```python
from build123d import *

# Parameters (mm, degrees)
BOSS_EXTRUDE1_DEPTH = 2.5
FILLET1_R           = 6.35


with BuildPart() as part:
    # Sketch1 → Boss-Extrude1 (new, symmetric)
    with BuildSketch(Plane.XY):
        Polygon((-63.5, 0), (-57.15, 25.4), (63.5, 25.4), (63.5, -25.4), (-63.5, -25.4), align=None)
    extrude(amount=BOSS_EXTRUDE1_DEPTH, both=True)

    # Fillet1
    fillet1_edges = [part.edges().sort_by_distance(p)[0] for p in [
        (63.5, -25.4, 0),
        (-63.5, -25.4, 0),
        (-63.5, 0, 0),
        (-57.15, 25.4, 0),
        (63.5, 25.4, 0),
    ]]
    fillet(fillet1_edges, radius=FILLET1_R)


solid = part.part
```
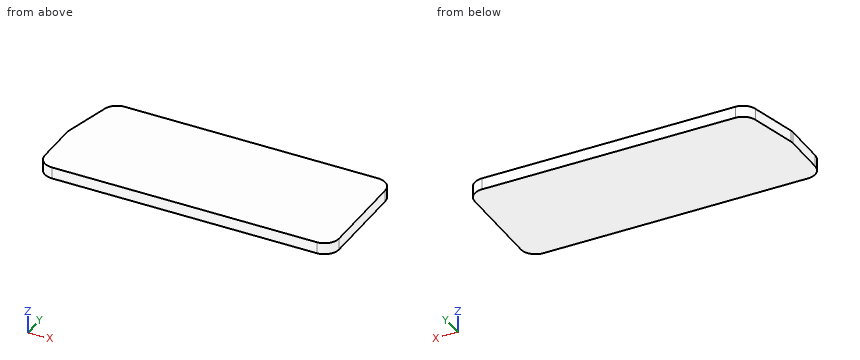
Could you check a few things on this model? Use its own coordinates, in mm. Coordinates: 2 decimals unless noted, no trailing zeros. Write each loop counter-clockwise with the first axis right and the second up, starting at its lowest first coordinate (ties: lowest second). Pieces come first, ordered by that corner, then holes. Notation, with made-up numbers: M -14,30.5 L 45,30.5 A15 cw 45,55.5 Z; hole C -8.75,-21 d10. An arc over 180 degrees is marked long. Answer as CSV lines item,"result". Start each with the question number.
1) Please list where these lines run through material, in increasing order: line 1 (X direction, y = 9.5, z = -0.05) (3 decimals); line 2 (X direction, y = 14, z = 1.75); line 3 (Y direction, x = -57.5, z = -0.7). Write a range as from..to.
2) I want a section at C-C, the plane y = 15.5. Please give me the cut outline in (x, z) (3 decimals).
3) I want a section at B-B, the plane y = 9. Please give me the cut outline in (x, z).
4) For P1, Ø1.5, axis at y = 10, z = -2, coming from the -X side, with a flat end and sliding along its axis, tell me the tip position at first contact or that it passes through.
5) I want a section at A-A, the plane z = 1.75. Please give me the cut outline in (x, y), and give its area (3 significant figures).
Data:
1,line 1,"x = -61.125..63.5"
1,line 2,"x = -60..63.5"
1,line 3,"y = -25.39..22.54"
2,outline,"M -59.625,-2.5 L 63.5,-2.5 L 63.5,2.5 L -59.625,2.5 Z"
3,outline,"M -61.25,-2.5 L 63.5,-2.5 L 63.5,2.5 L -61.25,2.5 Z"
4,P1,"stops at x = -61.19"
5,outline,"M -63.5,-19.05 A6.35 ccw -57.15,-25.4 L 57.15,-25.4 A6.35 ccw 63.5,-19.05 L 63.5,19.05 A6.35 ccw 57.15,25.4 L -52.19,25.4 A6.35 ccw -58.35,20.59 L -63.31,0.76 A6.35 ccw -63.5,-0.78 Z"
5,area,"6,340 mm^2"
